from build123d import *

# Parameters (mm, degrees)
SKETCH1_W           = 22
SKETCH1_H           = 140
BOSS_EXTRUDE1_DEPTH = 10
CHAMFER1_SIZE       = 2
SKETCH2_R           = 3
CUT_EXTRUDE1_DEPTH  = 11


with BuildPart() as part:
    # Sketch1 → Boss-Extrude1 (new body)
    with BuildSketch(Plane.XY):
        Rectangle(SKETCH1_W, SKETCH1_H)
    extrude(amount=BOSS_EXTRUDE1_DEPTH)

    # Chamfer1
    chamfer1_edges = [part.edges().sort_by_distance(p)[0] for p in [
        (11, 0, 0),
        (11, 0, 10),
    ]]
    chamfer(chamfer1_edges, length=CHAMFER1_SIZE)

    # Sketch2 → Cut-Extrude1 (cut, through all)
    with BuildSketch(Plane.XY.offset(10)):
        with Locations((-5, 55)):
            Circle(SKETCH2_R)
        with Locations((-5, 0)):
            Circle(SKETCH2_R)
        with Locations((-5, -55)):
            Circle(SKETCH2_R)
    extrude(amount=-CUT_EXTRUDE1_DEPTH, mode=Mode.SUBTRACT)


solid = part.part
Design review of the part built by this model. Coordinates are the model's own, in mm. Round coordinates to 2 decimals unless told otherwise and drop trailing zeros. Write each loop counter-clockwise with the first axis right and the second up, starting at its lowest first coordinate (ties: lowest second). Pieces come first, ordered by that corner, then holes. Notation, with made-up numbers: M 61,16.5 L 81,16.5 A16 ccw 81,28.5 Z; hole C -6.5,41 d6. An arc over 180 degrees is marked long. One line per item, written item: value. Start each with the question number.
1. Take a section at C-C on z = 6.5. State the section outline as (x, y) points.
2. Draft analysis for pull direction X (two halves, no side actions). For faces 1 (the face through (-5, 58, 5)), 2 (the face through (-11, -1, 5)), 3 (the face through (-1, 1, 0)), state which applies: pulls with the +X half, pulls with the -X half, needs draft (parallel to the pull), parting line crosses it, or undercut.
3. Take a section at A-A on y = 0. State the section outline as (x, z) points.
4. Take a section at B-B on x = -5.25. State the section outline as (y, z) points.
5. Clearance check with a flat-ended pin moving along its axis: P1, Ø9.5, axis at x = -5, y = 0, coming from the +Z side. State where the tip first meets the part, or that it passes through.
6. Take a section at D-D on y = 37. State the section outline as (x, z) points.
7. To check wall thickness, follow probe 1 along Y at (x, z) = (-3, 1.75); probe 2 along Y at (x, z) = (-6, 3.5); probe 3 along X at (y, z) = (-51, 1). State the ranges of each line that lie inside material, in increasing order. Write a range as from..to.
Computed:
1. outline: M -11,-70 L 11,-70 L 11,70 L -11,70 Z; hole C -5,-55 d6; hole C -5,0 d6; hole C -5,55 d6
2. face 1: undercut
2. face 2: pulls with the -X half
2. face 3: needs draft
3. outline: M -11,0 L -8,0 L -8,10 L -11,10 Z; M -2,0 L 9,0 L 11,2 L 11,8 L 9,10 L -2,10 Z
4. outline: M -70,0 L -57.99,0 L -57.99,10 L -70,10 Z; M -52.01,0 L -2.99,0 L -2.99,10 L -52.01,10 Z; M 2.99,0 L 52.01,0 L 52.01,10 L 2.99,10 Z; M 57.99,0 L 70,0 L 70,10 L 57.99,10 Z
5. P1: stops at z = 10
6. outline: M -11,0 L 9,0 L 11,2 L 11,8 L 9,10 L -11,10 Z
7. probe 1: y = -70..-57.24, -52.76..-2.24, 2.24..52.76, 57.24..70
7. probe 2: y = -70..-57.83, -52.17..-2.83, 2.83..52.17, 57.83..70
7. probe 3: x = -11..10
